from build123d import *

# Parameters (mm, degrees)
SKETCH_1_W          = 46
SKETCH_1_H          = 40
EXTRUDE_1_DEPTH     = 15
SKETCH_2_R          = 5
CUT_EXTRUDE_1_DEPTH = 43.766809561
SKETCH_4_W          = 14
SKETCH_4_H          = 3
CUT_EXTRUDE_2_DEPTH = 53.354560451
FILLET_3_R          = 3
FILLET_8_R          = 3
CUT_EXTRUDE_3_DEPTH = 53.354560451


with BuildPart() as part:
    # 草圖1 → 填料-伸長1 (new, symmetric)
    with BuildSketch(Plane.XY):
        Rectangle(SKETCH_1_W, SKETCH_1_H)
    extrude(amount=EXTRUDE_1_DEPTH, both=True)

    # 草圖2 → 除料-伸長1 (cut, through all)
    with BuildSketch(Plane.XY.offset(15)):
        with Locations((0, 10)):
            Circle(SKETCH_2_R)
    extrude(amount=-CUT_EXTRUDE_1_DEPTH, mode=Mode.SUBTRACT)

    # 草圖4 → 除料-伸長2 (cut, through all)
    with BuildSketch(Plane(origin=(23, 0, 0), x_dir=(0, 0, -1), z_dir=(1, 0, 0))):
        with Locations((0, -18.5)):
            Rectangle(SKETCH_4_W, SKETCH_4_H)
    extrude(amount=-CUT_EXTRUDE_2_DEPTH, mode=Mode.SUBTRACT)

    # 圓角3
    fillet_3_edges = [part.edges().sort_by_distance(p)[0] for p in [
        (0, -17, 7),
    ]]
    fillet(fillet_3_edges, radius=FILLET_3_R - 0.0001)  # a hair under: the kernel refuses the full size

    # 圓角8
    fillet_8_edges = [part.edges().sort_by_distance(p)[0] for p in [
        (0, -17, -7),
    ]]
    fillet(fillet_8_edges, radius=FILLET_8_R - 0.0001)  # a hair under: the kernel refuses the full size

    # 草圖5 → 除料-伸長3 (cut, through all)
    with BuildSketch(Plane(origin=(23, 0, 0), x_dir=(0, 0, -1), z_dir=(1, 0, 0))):
        Polygon((-5, 0), (5, 20), (-5, 20), (-15, 20), (-15, 0), align=None)
    extrude(amount=-CUT_EXTRUDE_3_DEPTH, mode=Mode.SUBTRACT)


solid = part.part
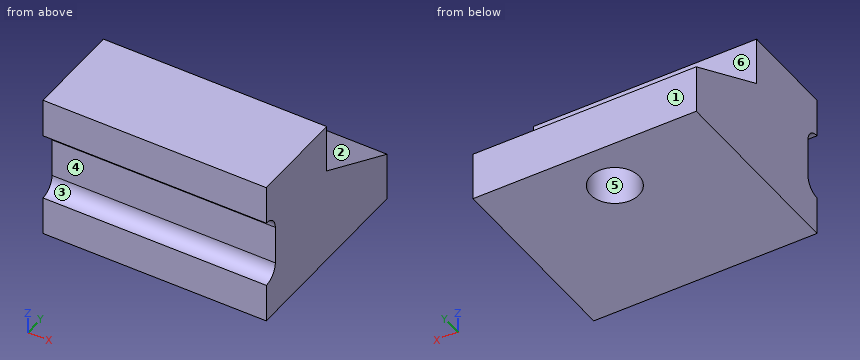
Work out the finished part from the listing and answer in its coordinate system (mm). Face numbers are marked on the shaded views. A direction names the side the tool comes from. Round coordinates to 2 decimals unless told otherwise and drop trailing zeros. Write each loop counter-clockwise with the first axis right and the second up, starting at its lowest first coordinate (ties: lowest second). Pieces come first, ordered by that corner, then holes. Notation, with made-up numbers: (-14.5, 54) - (-1.5, 54) arc R26 ccw to (-1.5, 86) - close; hole circle Ø8 at (75, 77). An arc over 180 degrees is marked (long way). Answer in a Markdown table with one row per item. Add a question column.
1. For the marked faces 4, 5 and 6, determine the directions among +Z, -Z, +X, -X, +Y, -Y from which every point of the face is accessible in a straight line to the end or side of a thin tool.
2. A cutting plane is placed at D-D, the plane z = 10. Determine the outline of the cut face in (x, y), and give its area (3 significant figures).
3. Given pin 1 (3 mm diameter, centred on x = -10, z = 3, fed in from -Y); pin 2 (9 mm diameter, centred on x = -8.5, z = -2, fed in from -Y); pin 3 (12 mm diameter, centred on x = 9, y = 1.5, fed in from +Z); pin 4 (9 mm diameter, centred on x = 0, y = 10, fed in from -Z), each flat-ended and moving along its own axis, determine where each tip first touches the part or whether it passes through.
4. The mould has two halves that part along Z. Classify the marked faces 1, 2 and 3: +Z half, -Z half, draft (parallel to the pull), parting line (faces both ways), or undercut.
5. Find the intervals of material crossed by line 1 along X through (y, z) = (10, -9.5); line 2 along Y through (x, z) = (0, -7.5); line 3 along Y through (x, z) = (0, -2.75), in increasing order. Write a range as from..to.
6. A cutting plane is placed at A-A, the plane y = 10. Determine the outline of the cut face in (x, z).
Worked out:
| question | item | result |
|---|---|---|
| 1 | face 4 | +X, -X, -Y |
| 1 | face 5 | +Z, -Z |
| 1 | face 6 | +Z, +X, -X, +Y |
| 2 | outline | (-23, -20) - (23, -20) - (23, 0) - (-23, 0) - close |
| 2 | area | 920 mm^2 |
| 3 | pin 1 | y = -17.04 |
| 3 | pin 2 | y = -18.34 |
| 3 | pin 3 | z = 15 |
| 3 | pin 4 | through |
| 4 | face 1 | draft |
| 4 | face 2 | +Z half |
| 4 | face 3 | undercut |
| 5 | line 1 | -23..-5, 5..23 |
| 5 | line 2 | -20..5, 15..20 |
| 5 | line 3 | -17..5, 15..15.5 |
| 6 | outline | (-23, -15) - (-5, -15) - (-5, 0) - (-23, 0) - close; (5, -15) - (23, -15) - (23, 0) - (5, 0) - close |
